from build123d import *

# Parameters (mm, degrees)
EXTRUDE_1_DEPTH              = 3
CUT_EXTRUDE_1_REACH          = 217.134
HOLE_WIZARD_M2_2_D           = 2.4
HOLE_WIZARD_M2_2_CBORE_D     = 4.4
HOLE_WIZARD_M2_2_CBORE_DEPTH = 2
CUT_EXTRUDE_2_REACH          = 217.134
HOLE_WIZARD_M2_3_D           = 2.4
HOLE_WIZARD_M2_3_CBORE_D     = 4.4
HOLE_WIZARD_M2_3_CBORE_DEPTH = 2
MIRROR_7_COPY_1_REACH        = 217.134
MIRROR_7_COPY_2_D            = 2.4
MIRROR_7_COPY_2_CBORE_D      = 4.4
MIRROR_7_COPY_2_CBORE_DEPTH  = 2
CUT_EXTRUDE_3_REACH          = 217.134
SKETCH_18_W                  = 20
SKETCH_18_H                  = 10
HOLE_WIZARD_M2_4_D           = 2.4
HOLE_WIZARD_M2_4_CBORE_D     = 4.4
HOLE_WIZARD_M2_4_CBORE_DEPTH = 2
HOLE_WIZARD_M2_5_D           = 2.4
HOLE_WIZARD_M2_5_CBORE_D     = 4.4
HOLE_WIZARD_M2_5_CBORE_DEPTH = 2
HOLE_WIZARD_M2_6_D           = 2.4
HOLE_WIZARD_M2_6_CBORE_D     = 4.4
HOLE_WIZARD_M2_6_CBORE_DEPTH = 2
SKETCH_24_W                  = 20
SKETCH_24_H                  = 56
CUT_EXTRUDE_4_DEPTH          = 10
HOLE_WIZARD_M2_7_D           = 2.4
HOLE_WIZARD_M2_7_CBORE_D     = 4.4
HOLE_WIZARD_M2_7_CBORE_DEPTH = 2
SKETCH_26_OUTSIDE_W          = 390.69
SKETCH_26_OUTSIDE_H          = 393.83
SKETCH_26_OUTSIDE_W_2        = 112.890872965
SKETCH_26_OUTSIDE_H_2        = 124.890872965
CUT_EXTRUDE_5_DEPTH          = 10


with BuildPart() as part:
    # 草图1 → 凸台-拉伸1 (new body)
    with BuildSketch(Plane(origin=(0, 0, 0), x_dir=(1, 0, 0), z_dir=(0, 1, 0))):
        Polygon((-45.715728753, 114), (45.715728753, 114), (84.606601718, 152.890872965), (91.67766953, 152.890872965), (112.890872965, 131.67766953), (112.890872965, 124.606601718), (74, 85.715728753), (74, 30), (91.320508076, 20), (146.320508076, 20), (151.320508076, 15), (151.320508076, -15), (146.320508076, -20), (91.320508076, -20), (74, -30), (74, -85.715728753), (112.890872965, -124.606601718), (112.890872965, -131.67766953), (91.67766953, -152.890872965), (84.606601718, -152.890872965), (45.715728753, -114), (-45.715728753, -114), (-84.606601718, -152.890872965), (-91.67766953, -152.890872965), (-112.890872965, -131.67766953), (-112.890872965, -124.606601718), (-74, -85.715728753), (-74, -30), (-91.320508076, -20), (-146.320508076, -20), (-151.320508076, -15), (-151.320508076, 15), (-146.320508076, 20), (-91.320508076, 20), (-74, 30), (-74, 85.715728753), (-112.890872965, 124.606601718), (-112.890872965, 131.67766953), (-91.67766953, 152.890872965), (-84.606601718, 152.890872965), align=None)
    extrude(amount=EXTRUDE_1_DEPTH)

    # 草图2 → 切除-拉伸1 (cut, up to next)
    with BuildSketch(Plane(origin=(0, 3, 0), x_dir=(1, 0, 0), z_dir=(0, 1, 0)), mode=Mode.PRIVATE) as cut_extrude_1_sk1:
        with BuildLine():
            Line((103.820508076, -10), (103.820508076, 10))
            Line((103.820508076, 10), (142.820508076, 10))
            ThreePointArc((142.820508076, 10), (144.234721638, 9.414213562), (144.820508076, 8))
            Line((144.820508076, 8), (144.820508076, -8))
            ThreePointArc((144.820508076, -8), (144.234721638, -9.414213562), (142.820508076, -10))
            Line((142.820508076, -10), (103.820508076, -10))
        make_face()
    cut_extrude_1_tool1 = extrude(cut_extrude_1_sk1.sketch, amount=-CUT_EXTRUDE_1_REACH, mode=Mode.PRIVATE) & part.part
    cut_extrude_1 = cut_extrude_1_tool1.solids().sort_by_distance((124.278435, 3, 0))[0]
    add(cut_extrude_1, mode=Mode.SUBTRACT)

    # M2 凹头盖螺钉的柱形沉头孔2 (through all)
    with Locations(Plane(origin=(100.320508076, 3, -8), x_dir=(0, 0, 1), z_dir=(0, 1, 0))):
        with Locations((0, 0), (-5.5, 5.25), (-5.5, 13.25), (-5.5, 21.25), (-5.5, 29.25), (16, 0), (21.5, 5.25), (21.5, 13.25), (21.5, 21.25), (21.5, 29.25)):
            hole_wizard_m2_2 = CounterBoreHole(HOLE_WIZARD_M2_2_D / 2, HOLE_WIZARD_M2_2_CBORE_D / 2, HOLE_WIZARD_M2_2_CBORE_DEPTH)

    # 草图10 → 切除-拉伸2 (cut, up to next)
    with BuildSketch(Plane(origin=(0, 3, 0), x_dir=(1, 0, 0), z_dir=(0, 1, 0)), mode=Mode.PRIVATE) as cut_extrude_2_sk1:
        with BuildLine():
            Line((75.767766953, 101.625631329), (61.625631329, 115.767766953))
            Line((61.625631329, 115.767766953), (79.916185958, 134.058321582))
            Line((79.916185958, 134.058321582), (89.202795796, 143.344931419))
            ThreePointArc((89.202795796, 143.344931419), (90.617009358, 143.930717857), (92.03122292, 143.344931419))
            Line((92.03122292, 143.344931419), (97.68807717, 137.68807717))
            Line((97.68807717, 137.68807717), (103.344931419, 132.03122292))
            ThreePointArc((103.344931419, 132.03122292), (103.930717857, 130.617009358), (103.344931419, 129.202795796))
            Line((103.344931419, 129.202795796), (94.058321582, 119.916185958))
            Line((94.058321582, 119.916185958), (75.767766953, 101.625631329))
        make_face()
    cut_extrude_2_tool1 = extrude(cut_extrude_2_sk1.sketch, amount=-CUT_EXTRUDE_2_REACH, mode=Mode.PRIVATE) & part.part
    cut_extrude_2 = cut_extrude_2_tool1.solids().sort_by_distance((83.162638, 3, -123.162638))[0]
    add(cut_extrude_2, mode=Mode.SUBTRACT)

    # M2 凹头盖螺钉的柱形沉头孔3 (through all)
    with Locations(Plane(origin=(60.388194462, 3, -119.480077554), x_dir=(0, 0, 1), z_dir=(0, 1, 0))):
        with Locations((0, 0), (-5.65685425, 5.65685425), (-11.313708499, 11.313708499), (-16.970562749, 16.970562749), (7.601397898, 0.176776695), (18.915106397, 11.490485194), (19.091883092, 19.091883092), (13.435028842, 24.748737342), (7.778174593, 30.405591591), (2.121320343, 36.062445841)):
            hole_wizard_m2_3 = CounterBoreHole(HOLE_WIZARD_M2_3_D / 2, HOLE_WIZARD_M2_3_CBORE_D / 2, HOLE_WIZARD_M2_3_CBORE_DEPTH)

    # 镜向5: 切除-拉伸1, M2 凹头盖螺钉的柱形沉头孔2 across plane
    add(cut_extrude_1.mirror(Plane(origin=(0, 0, 0), x_dir=(0, 0, 1), z_dir=(1, 0, 0))), mode=Mode.SUBTRACT)
    add(hole_wizard_m2_2.mirror(Plane(origin=(0, 0, 0), x_dir=(0, 0, 1), z_dir=(1, 0, 0))), mode=Mode.SUBTRACT)

    # 镜向6: 切除-拉伸2, M2 凹头盖螺钉的柱形沉头孔3 across plane
    add(cut_extrude_2.mirror(Plane(origin=(0, 0, 0), x_dir=(0, 0, 1), z_dir=(1, 0, 0))), mode=Mode.SUBTRACT)
    add(hole_wizard_m2_3.mirror(Plane(origin=(0, 0, 0), x_dir=(0, 0, 1), z_dir=(1, 0, 0))), mode=Mode.SUBTRACT)

    # 镜向7: 切除-拉伸2, M2 凹头盖螺钉的柱形沉头孔3 across plane
    add(cut_extrude_2.mirror(Plane.XY), mode=Mode.SUBTRACT)
    add(hole_wizard_m2_3.mirror(Plane.XY), mode=Mode.SUBTRACT)

    # 镜向7 copy 1 sketch → 镜向7 copy 1 (cut, up to next)
    with BuildSketch(Plane(origin=(0, 3, 0), x_dir=(-1, 0, 0), z_dir=(0, 1, 0)), mode=Mode.PRIVATE) as mirror_7_copy_1_sk1:
        with BuildLine():
            Line((75.767766953, 101.625631329), (61.625631329, 115.767766953))
            Line((61.625631329, 115.767766953), (79.916185958, 134.058321582))
            Line((79.916185958, 134.058321582), (89.202795796, 143.344931419))
            ThreePointArc((89.202795796, 143.344931419), (90.617009358, 143.930717857), (92.03122292, 143.344931419))
            Line((92.03122292, 143.344931419), (97.68807717, 137.68807717))
            Line((97.68807717, 137.68807717), (103.344931419, 132.03122292))
            ThreePointArc((103.344931419, 132.03122292), (103.930717857, 130.617009358), (103.344931419, 129.202795796))
            Line((103.344931419, 129.202795796), (94.058321582, 119.916185958))
            Line((94.058321582, 119.916185958), (75.767766953, 101.625631329))
        make_face()
    mirror_7_copy_1_tool1 = extrude(mirror_7_copy_1_sk1.sketch, amount=-MIRROR_7_COPY_1_REACH, mode=Mode.PRIVATE) & part.part
    add(mirror_7_copy_1_tool1.solids().sort_by_distance((-83.162638, 3, 123.162638))[0], mode=Mode.SUBTRACT)

    # 镜向7 copy 2 (through all)
    with Locations(Plane(origin=(-60.388194462, 3, 119.480077554), x_dir=(0, 0, -1), z_dir=(0, 1, 0))):
        with Locations((0, 0), (-5.65685425, 5.65685425), (-11.313708499, 11.313708499), (-16.970562749, 16.970562749), (7.601397898, 0.176776695), (18.915106397, 11.490485194), (19.091883092, 19.091883092), (13.435028842, 24.748737342), (7.778174593, 30.405591591), (2.121320343, 36.062445841)):
            CounterBoreHole(MIRROR_7_COPY_2_D / 2, MIRROR_7_COPY_2_CBORE_D / 2, MIRROR_7_COPY_2_CBORE_DEPTH)

    # 草图18 → 切除-拉伸3 (cut, up to next)
    with BuildSketch(Plane(origin=(0, 3, 0), x_dir=(1, 0, 0), z_dir=(0, 1, 0)), mode=Mode.PRIVATE) as cut_extrude_3_sk1:
        Polygon((-60, -28), (-15, -28), (-15, -63), (-60, -83), align=None)
    cut_extrude_3_tool1 = extrude(cut_extrude_3_sk1.sketch, amount=-CUT_EXTRUDE_3_REACH, mode=Mode.PRIVATE) & part.part
    # 草图18 → 切除-拉伸3 (cut, up to next)
    with BuildSketch(Plane(origin=(0, 3, 0), x_dir=(1, 0, 0), z_dir=(0, 1, 0)), mode=Mode.PRIVATE) as cut_extrude_3_sk2:
        with Locations((20, -99)):
            Rectangle(SKETCH_18_W, SKETCH_18_H)
    cut_extrude_3_tool2 = extrude(cut_extrude_3_sk2.sketch, amount=-CUT_EXTRUDE_3_REACH, mode=Mode.PRIVATE) & part.part
    # 草图18 → 切除-拉伸3 (cut, up to next)
    with BuildSketch(Plane(origin=(0, 3, 0), x_dir=(1, 0, 0), z_dir=(0, 1, 0)), mode=Mode.PRIVATE) as cut_extrude_3_sk3:
        with Locations((-20, -99)):
            Rectangle(SKETCH_18_W, SKETCH_18_H)
    cut_extrude_3_tool3 = extrude(cut_extrude_3_sk3.sketch, amount=-CUT_EXTRUDE_3_REACH, mode=Mode.PRIVATE) & part.part
    # 草图18 → 切除-拉伸3 (cut, up to next)
    with BuildSketch(Plane(origin=(0, 3, 0), x_dir=(1, 0, 0), z_dir=(0, 1, 0)), mode=Mode.PRIVATE) as cut_extrude_3_sk4:
        Polygon((15, -63), (60, -83), (60, -28), (15, -28), align=None)
    cut_extrude_3_tool4 = extrude(cut_extrude_3_sk4.sketch, amount=-CUT_EXTRUDE_3_REACH, mode=Mode.PRIVATE) & part.part
    # 草图18 → 切除-拉伸3 (cut, up to next)
    with BuildSketch(Plane(origin=(0, 3, 0), x_dir=(1, 0, 0), z_dir=(0, 1, 0)), mode=Mode.PRIVATE) as cut_extrude_3_sk5:
        with Locations((-20, 99)):
            Rectangle(SKETCH_18_W, SKETCH_18_H)
    cut_extrude_3_tool5 = extrude(cut_extrude_3_sk5.sketch, amount=-CUT_EXTRUDE_3_REACH, mode=Mode.PRIVATE) & part.part
    # 草图18 → 切除-拉伸3 (cut, up to next)
    with BuildSketch(Plane(origin=(0, 3, 0), x_dir=(1, 0, 0), z_dir=(0, 1, 0)), mode=Mode.PRIVATE) as cut_extrude_3_sk6:
        with Locations((20, 99)):
            Rectangle(SKETCH_18_W, SKETCH_18_H)
    cut_extrude_3_tool6 = extrude(cut_extrude_3_sk6.sketch, amount=-CUT_EXTRUDE_3_REACH, mode=Mode.PRIVATE) & part.part
    # 草图18 → 切除-拉伸3 (cut, up to next)
    with BuildSketch(Plane(origin=(0, 3, 0), x_dir=(1, 0, 0), z_dir=(0, 1, 0)), mode=Mode.PRIVATE) as cut_extrude_3_sk7:
        Polygon((15, 63), (60, 83), (60, 28), (15, 28), align=None)
    cut_extrude_3_tool7 = extrude(cut_extrude_3_sk7.sketch, amount=-CUT_EXTRUDE_3_REACH, mode=Mode.PRIVATE) & part.part
    # 草图18 → 切除-拉伸3 (cut, up to next)
    with BuildSketch(Plane(origin=(0, 3, 0), x_dir=(1, 0, 0), z_dir=(0, 1, 0)), mode=Mode.PRIVATE) as cut_extrude_3_sk8:
        Polygon((-15, 28), (-15, 63), (-60, 83), (-60, 28), align=None)
    cut_extrude_3_tool8 = extrude(cut_extrude_3_sk8.sketch, amount=-CUT_EXTRUDE_3_REACH, mode=Mode.PRIVATE) & part.part
    add(cut_extrude_3_tool1.solids().sort_by_distance((-39.166667, 3, 50.87037))[0], mode=Mode.SUBTRACT)
    add(cut_extrude_3_tool2.solids().sort_by_distance((20, 3, 99))[0], mode=Mode.SUBTRACT)
    add(cut_extrude_3_tool3.solids().sort_by_distance((-20, 3, 99))[0], mode=Mode.SUBTRACT)
    add(cut_extrude_3_tool4.solids().sort_by_distance((39.166667, 3, 50.87037))[0], mode=Mode.SUBTRACT)
    add(cut_extrude_3_tool5.solids().sort_by_distance((-20, 3, -99))[0], mode=Mode.SUBTRACT)
    add(cut_extrude_3_tool6.solids().sort_by_distance((20, 3, -99))[0], mode=Mode.SUBTRACT)
    add(cut_extrude_3_tool7.solids().sort_by_distance((39.166667, 3, -50.87037))[0], mode=Mode.SUBTRACT)
    add(cut_extrude_3_tool8.solids().sort_by_distance((-39.166667, 3, -50.87037))[0], mode=Mode.SUBTRACT)

    # M2 凹头盖螺钉的柱形沉头孔4 (through all)
    with Locations(Plane(origin=(-20, 3, 109), x_dir=(0, 0, 1), z_dir=(0, 1, 0))):
        with Locations((0, 0), (0, 40), (-218, 0), (-218, 40)):
            CounterBoreHole(HOLE_WIZARD_M2_4_D / 2, HOLE_WIZARD_M2_4_CBORE_D / 2, HOLE_WIZARD_M2_4_CBORE_DEPTH)

    # M2 凹头盖螺钉的柱形沉头孔5 (through all)
    with Locations(Plane(origin=(-69, 3, -40), x_dir=(0, 0, 1), z_dir=(0, 1, 0))):
        with Locations((0, 0), (0, 138)):
            hole_wizard_m2_5 = CounterBoreHole(HOLE_WIZARD_M2_5_D / 2, HOLE_WIZARD_M2_5_CBORE_D / 2, HOLE_WIZARD_M2_5_CBORE_DEPTH)

    # 镜向8: M2 凹头盖螺钉的柱形沉头孔5 across plane
    add(hole_wizard_m2_5.mirror(Plane.XY), mode=Mode.SUBTRACT)

    # M2 凹头盖螺钉的柱形沉头孔6 (through all)
    with Locations(Plane(origin=(-69, 3, 0), x_dir=(0, 0, 1), z_dir=(0, 1, 0))):
        with Locations((0, 0), (0, 138)):
            CounterBoreHole(HOLE_WIZARD_M2_6_D / 2, HOLE_WIZARD_M2_6_CBORE_D / 2, HOLE_WIZARD_M2_6_CBORE_DEPTH)

    # 草图24 → 切除-拉伸4 (cut)
    with BuildSketch(Plane(origin=(0, 3, 0), x_dir=(1, 0, 0), z_dir=(0, 1, 0))):
        Rectangle(SKETCH_24_W, SKETCH_24_H)
    extrude(amount=-CUT_EXTRUDE_4_DEPTH, mode=Mode.SUBTRACT)

    # M2 凹头盖螺钉的柱形沉头孔7 (through all)
    with Locations(Plane(origin=(-20, 3, 0), x_dir=(0, 0, 1), z_dir=(0, 1, 0))):
        with Locations((0, 0), (0, 40)):
            CounterBoreHole(HOLE_WIZARD_M2_7_D / 2, HOLE_WIZARD_M2_7_CBORE_D / 2, HOLE_WIZARD_M2_7_CBORE_DEPTH)

    # 草图26 outside → 切除-拉伸5 (cut)
    with BuildSketch(Plane(origin=(0, 3, 0), x_dir=(1, 0, 0), z_dir=(0, 1, 0))):
        Rectangle(SKETCH_26_OUTSIDE_W, SKETCH_26_OUTSIDE_H)
        with Locations((-56.445436483, 90.445436482)):
            Rectangle(SKETCH_26_OUTSIDE_W_2, SKETCH_26_OUTSIDE_H_2, mode=Mode.SUBTRACT)
    extrude(amount=-CUT_EXTRUDE_5_DEPTH, mode=Mode.SUBTRACT)


solid = part.part
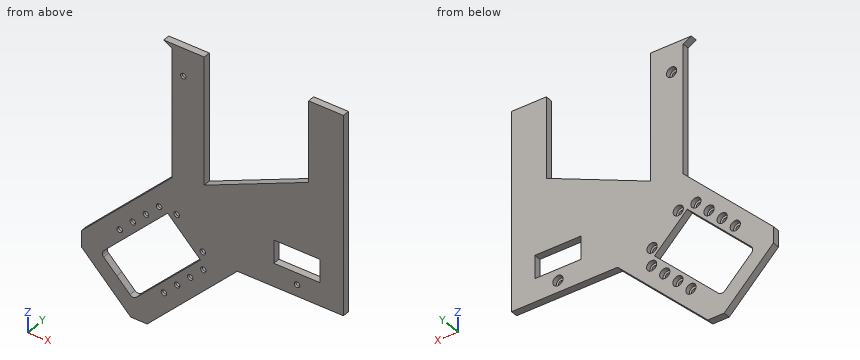
Geometry: final body of the model. Coordinates: model frame, mm. Coordinates: 2 decimals unless noted, no trailing zeros. Order: outer loops, then holes, each group sorted by start corner. A loop starts at its lowest first (then second) coordinate and runs counter-clockwise, first axis right, second up.
(1) First-contact query: pin 1 (2 mm diameter, centred on x = -97, z = -116.5, fed in from +Y); pin 2 (1.5 mm diameter, centred on y = 2, z = -98, fed in from -X); pin 3 (1.5 mm diameter, centred on x = -38, y = 1.5, fed in from +Z); pin 4 (1.4 mm diameter, centred on x = -69, z = -40, fed in from -Y). Flat tips, straight axial feed; report the tip coordinate or a pass-through.
(2) Material intervals for probe 1 along X at (y, z) = (1.15, -44); probe 2 along X at (y, z) = (2.8, -100); probe 3 along Z at (x, y) = (-24.5, 1.6), sorted ascending.
(3) Section query C-C (x = -8). Return the cut outline in (y, z), plus the area to 3 significant figures.
(4) Section query A-A (z = -67.5). Return the cut outline in (x, y) (3 decimals).
(5) Section query B-B (y = 2.4). State how many separate pieces and enclosed holes the cut face has, plus the area to 3 significant figures.
Solution:
1. pin 1: stops at y = 1
1. pin 2: stops at x = -87.03
1. pin 3: stops at z = -72.89
1. pin 4: passes through
2. probe 1: x = -74 to -60, -15 to 0
2. probe 2: x = -88.28 to -81.65, -77.31 to -74, -69.75 to -30, -10 to 0
2. probe 3: z = -114 to -104, -94 to -67.22
3. outline: (0, -114) - (3, -114) - (3, -28) - (0, -28) - close
3. area: 258 mm2
4. outline: (-74, 0) - (-60, 0) - (-60, 3) - (-74, 3) - close; (-25.125, 0) - (0, 0) - (0, 3) - (-25.125, 3) - close
5. separate pieces: 1
5. enclosed holes: 14
5. area: 5,120 mm2
